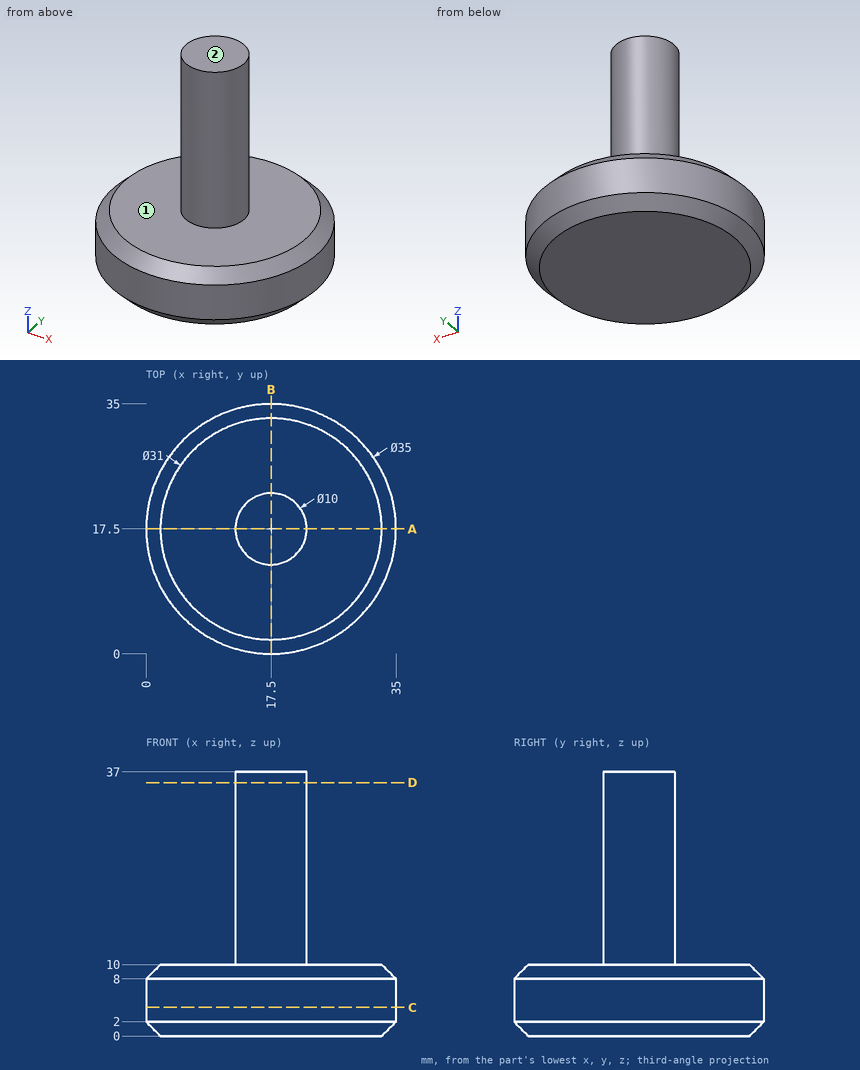
Geometry check sheet. Reference: drawing and pictorial views, mm from the part's lowest x, y, z. A direction names the side the tool comes from. Give positions to 0.01 mm unless a question says otherwise; leave off trailing zeros. Loops run counter-clockwise (first coordinate to the right, second up) from the corner with the lowest first, then second, coordinate; pieces in that order, holes last.
1. Section check A-A, the plane y = 17.5. Enter the section's corners in (x, z).
2. Set-up check for the marked faces 1 and 2: record each of +Z, -Z, +X, -X, +Y, -Y from which the full face is reachable in a straight line by a thin tool's end or side.
3. Thickness scan on line 1 (Z direction, x = 19, y = 28.5); line 2 (X direction, y = 17, z = 4.5); line 3 (Y direction, x = 17.5, z = 31.5). Record the ranges inside material, lowest first.
4. Section check D-D, the plane z = 35.5. Enter the section's corners in (x, y), then the cut area to 3 significant figures.
5. Go/stop test with flat-tipped pins: pin 1 Ø2 at (x, y) = (20, 4) entering from -Z; pin 2 Ø1 at (x, y) = (5.5, 27.5) entering from +Z; pin 3 Ø8 at (y, z) = (22.5, 20.5) entering from +X; pin 4 Ø8 at (y, z) = (4.5, 7) entering from -X. Record where each tip stops, or that it passes through.
6. Section check C-C, the plane z = 4. Enter the section's corners in (x, y), then the cut area to 3 significant figures.
Geometry says:
1. outline: (0, 2) - (2, 0) - (33, 0) - (35, 2) - (35, 8) - (33, 10) - (22.5, 10) - (22.5, 37) - (12.5, 37) - (12.5, 10) - (2, 10) - (0, 8) - close
2. face 1: +Z
2. face 2: +Z, +X, -X, +Y, -Y
3. line 1: z = 0 to 10
3. line 2: x = 0.01 to 34.99
3. line 3: y = 12.5 to 22.5
4. outline: circle Ø10 at (17.5, 17.5)
4. area: 78.5 mm2
5. pin 1: stops at z = 0
5. pin 2: stops at z = 10
5. pin 3: stops at x = 22.4
5. pin 4: stops at x = 2.49
6. outline: circle Ø35 at (17.5, 17.5)
6. area: 962 mm2
